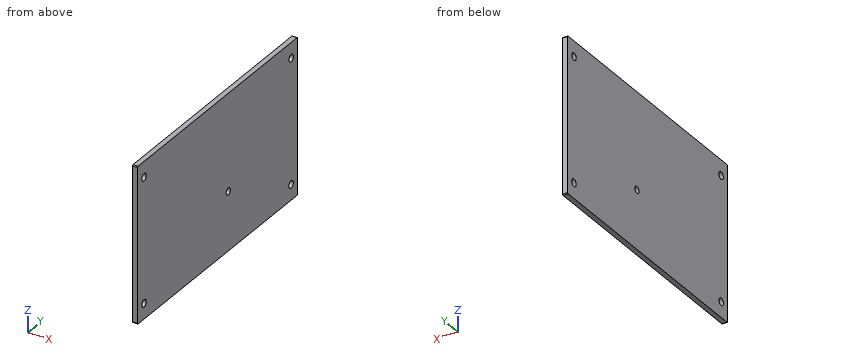
```python
from build123d import *

# Parameters (mm, degrees)
SKETCH1_W           = 90
SKETCH1_H           = 150
SKETCH1_R           = 1.925
SKETCH1_R_2         = 2.1
BOSS_EXTRUDE1_DEPTH = 3
FILLET1_R           = 0.5


with BuildPart() as part:
    # Sketch1 → Boss-Extrude1 (new body)
    with BuildSketch(Plane(origin=(0, 0, 0), x_dir=(0, 0, -1), z_dir=(1, 0, 0))):
        with Locations((45, -75)):
            Rectangle(SKETCH1_W, SKETCH1_H)
        with Locations((56, -65)):
            Circle(SKETCH1_R, mode=Mode.SUBTRACT)
        with Locations((9, -6)):
            Circle(SKETCH1_R_2, mode=Mode.SUBTRACT)
        with Locations(Location((81, -6, 0), (0, 0, 180))):
            Circle(SKETCH1_R_2, mode=Mode.SUBTRACT)
        with Locations((81, -144)):
            Circle(SKETCH1_R_2, mode=Mode.SUBTRACT)
        with Locations(Location((9, -144, 0), (0, 0, 180))):
            Circle(SKETCH1_R_2, mode=Mode.SUBTRACT)
    extrude(amount=BOSS_EXTRUDE1_DEPTH)

    # Fillet1
    fillet1_edges = [part.edges().sort_by_distance(p)[0] for p in [
        (1.5, 0, 0),
        (1.5, 0, -90),
        (1.5, -150, -90),
        (1.5, -150, 0),
    ]]
    fillet(fillet1_edges, radius=FILLET1_R)


solid = part.part
```
Check sheet for the modelled part. Datum: model origin and axes. Units: mm. Round coordinates to 2 decimals unless told otherwise and drop trailing zeros. Write each loop counter-clockwise with the first axis right and the second up, starting at its lowest first coordinate (ties: lowest second). Pieces come first, ordered by that corner, then holes. Notation, with made-up numbers: M 27,34.25 L 54,34.25 A7 cw 54,47.25 Z; hole C 52,-39 d3. An arc over 180 degrees is marked long. Write item = value, one per line. Start each with the question number.
1. Scan lines: line 1 (Z direction, x = 2.25, y = -144); line 2 (Y direction, x = 0.8, z = -9); line 3 (Y direction, x = 0.5, z = -10). Record each from-to range of solid material in increasing order. Write a range as [from, to].
2. Section check D-D, the plane z = -56. Record the cut outline in (x, y) (3 decimals), then the cut area to 3 significant figures.
3. Section check A-A, the plane z = -81. Record the cut outline in (x, y).
4. Section check B-B, the plane y = -65. Record the cut outline in (x, z) (3 decimals).
5. Section check C-C, the plane y = -6. Record the cut outline in (x, z).
Results found:
q1.line_1 = [-90, -83.1], [-78.9, -11.1], [-6.9, 0]
q1.line_2 = [-150, -146.1], [-141.9, -8.1], [-3.9, 0]
q1.line_3 = [-150, -145.85], [-142.15, -7.85], [-4.15, 0]
q2.outline = M 0,-150 L 3,-150 L 3,-66.925 L 0,-66.925 Z; M 0,-63.075 L 3,-63.075 L 3,0 L 0,0 Z
q2.area = 438 mm^2
q3.outline = M 0,-150 L 3,-150 L 3,-146.1 L 0,-146.1 Z; M 0,-141.9 L 3,-141.9 L 3,-8.1 L 0,-8.1 Z; M 0,-3.9 L 3,-3.9 L 3,0 L 0,0 Z
q4.outline = M 0,-90 L 3,-90 L 3,-57.925 L 0,-57.925 Z; M 0,-54.075 L 3,-54.075 L 3,0 L 0,0 Z
q5.outline = M 0,-90 L 3,-90 L 3,-83.1 L 0,-83.1 Z; M 0,-78.9 L 3,-78.9 L 3,-11.1 L 0,-11.1 Z; M 0,-6.9 L 3,-6.9 L 3,0 L 0,0 Z
